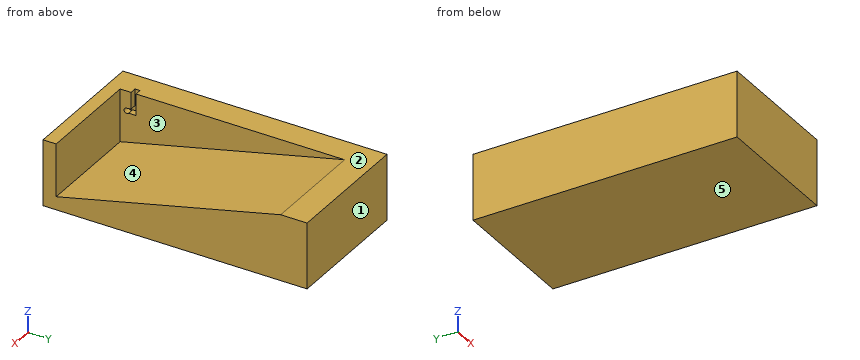
```python
from build123d import *

# Parameters (mm, degrees)
F0_W     = 20
F0_H     = 40
F1_DEPTH = 10
F3_DEPTH = 16
F5_DEPTH = 1


with BuildPart() as f1:
    # F0 (on Top) → F1 (new body)
    with BuildSketch(Plane.XY):
        with Locations((-10, 20)):
            Rectangle(F0_W, F0_H)
    extrude(amount=F1_DEPTH)

    # F2 (on face) → F3 (cut)
    with BuildSketch(Plane.YZ):
        Polygon((2, 2), (36, 10), (2, 10), align=None)
    extrude(amount=-F3_DEPTH, mode=Mode.SUBTRACT)

    # F4 (on face) → F5 (cut)
    with BuildSketch(Plane.YZ.offset(-16)):
        with BuildLine():
            Line((4.403491, 10), (3.653491, 10))
            Line((3.653491, 10), (3.653491, 7.472175))
            Line((3.653491, 7.472175), (2.957461, 7.397732))
            ThreePointArc((2.957461, 7.397732), (2.640655, 6.824299), (3.287773, 6.722175))
            Line((3.287773, 6.722175), (4.403491, 6.722175))
            Line((4.403491, 6.722175), (4.403491, 10))
        make_face()
    extrude(amount=-F5_DEPTH, mode=Mode.SUBTRACT)


solid = f1.part
```
Part model, mm, in its own coordinate system. Face numbers are marked on the shaded views. A direction names the side the tool comes from. Coordinates: 2 decimals unless noted, no trailing zeros. Loops run counter-clockwise (first coordinate to the right, second up) from the corner with the lowest first, then second, coordinate; pieces in that order, holes last. Notation, with made-up numbers: (68.5, -5) - (116.5, -5) arc R15 ccw to (116.5, 6) - close; hole circle Ø10 at (29.25, 13.5). An arc over 180 degrees is marked (long way). Write item = value, one per line. Start each with the question number.
Item 1: Flat gauge pin, fed straight in: pin 1 Ø1 at (x, y) = (-2, 13) entering from +Z. Where does the tip first touch, or does it go through?
Item 2: Cut at A-A, the plane x = -9.5. Give the cut face in (y, z).
Item 3: Mould opens along Y. For the marked faces 1, 2 and 3 say: released by +Y, released by -Y, zero draft, split by the parting line, or undercut.
Item 4: Cut at D-D, the plane z = 4.5. Give the cut face in (x, y) (3 decimals), and give its area (3 significant figures).
Item 5: Cut at B-B, the plane z = 8. Give the cut face in (x, y).
Item 6: 3-axis set-ups, long thin cutter, end or side, ignore diameter. For the marked faces 4 and 5: which of +Z, -Z, +X, -X, +Y, -Y reach the whole face in a straight line?
Item 7: Wall check: L1, parallel to Z at x = -16.4, y = 3; L2, parallel to Y at x = -16.6, z = 7; L3, parallel to X at y = 16, z = 6.5. Give the ranges that are in metal, low to high. Write a range as from..to.
Item 8: Cut at C-C, the plane y = 25. Give the cut face in (x, z).
The answers:
q1.pin_1 = 4.71
q2.outline = (0, 0) - (40, 0) - (40, 10) - (36, 10) - (2, 2) - (2, 10) - (0, 10) - close
q3.face_1 = released by +Y
q3.face_2 = zero draft
q3.face_3 = undercut
q4.outline = (-20, 0) - (0, 0) - (0, 2) - (-16, 2) - (-16, 12.625) - (0, 12.625) - (0, 40) - (-20, 40) - close
q4.area = 630 mm2
q5.outline = (-20, 0) - (0, 0) - (0, 2) - (-16, 2) - (-16, 3.65) - (-17, 3.65) - (-17, 4.4) - (-16, 4.4) - (-16, 27.5) - (0, 27.5) - (0, 40) - (-20, 40) - close
q6.face_4 = +Z, +X
q6.face_5 = -Z, +X, -X, +Y, -Y
q7.L1 = 0..6.6, 7.4..10
q7.L2 = 0..2.6, 4.4..40
q7.L3 = -20..-16
q8.outline = (-20, 0) - (0, 0) - (0, 7.41) - (-16, 7.41) - (-16, 10) - (-20, 10) - close
